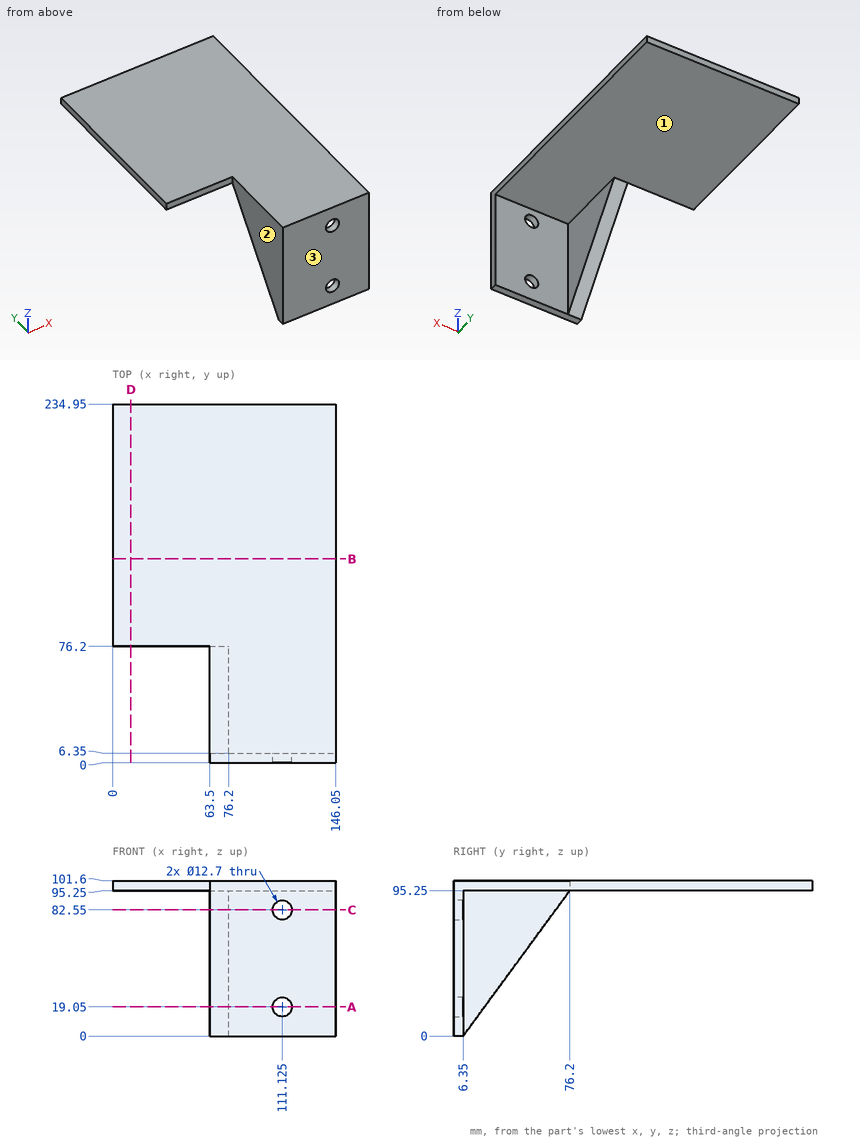
Geometry: see drawing. Coordinates: mm, zero at the bounding-box minimum. A direction names the side the tool comes from. Give positions to 0.01 mm unless a question says otherwise; leave off trailing zeros. Write each loop counter-clockwise with the first axis right and the second up, starting at its lowest first coordinate (ties: lowest second). Pieces come first, ordered by that corner, then holes. Notation, with made-up numbers: (84.5, 48.5) -> (131.5, 48.5) arc R10 cw to (131.5, 64.5) -> close; hole circle Ø10 at (15.25, 37.25). An arc over 180 degrees is marked (long way). Use one line per item in the form item = value. Start each with the question number.
1) Ray query, probe 1 along X at (y, z) = (1, 19); probe 2 along Z at (x, y) = (17, 101); probe 3 along Y at (x, z) = (26, 98.5). Return the intervals inside material, ascending. Write a range as from..to.
2) Set-up query: the marked faces 1, 2 and 3. Return all of +Z, -Z, +X, -X, +Y, -Y with unobstructed straight access to the full face (end or side cutting, diameter ignored); none if empty.
3) Section query D-D on x = 12. Return the cut outline in (y, z).
4) Section query C-C on z = 82.55. Return the cut outline in (x, y) (3 decimals).
5) Section query B-B on y = 133.5. Return the cut outline in (x, z).
6) Pin query (flat end, axial travel): pin 1 (2 mm diameter, centred on x = 123, y = 83, fed in from -Z); pin 2 (20.5 mm diameter, centred on x = 111.125, z = 19.05, fed in from +Y); pin 3 (21 mm diameter, centred on y = 54.5, z = 56.5, fed in from +X). Return the tip coordinate at first contact, or that it passes through.
7) Section query A-A on z = 19.05. Return the cut outline in (x, y) (3 decimals), then the cut area to 3 significant figures.
Outcome:
q1.probe_1 = 63.5..104.78, 117.47..146.05
q1.probe_2 = 95.25..101.6
q1.probe_3 = 76.2..234.95
q2.face_1 = -Z, +X, +Y
q2.face_2 = +Z, -Z, -X, -Y
q2.face_3 = +Z, -Z, +X, -X, -Y
q3.outline = (76.2, 95.25) -> (234.95, 95.25) -> (234.95, 101.6) -> (76.2, 101.6) -> close
q4.outline = (63.5, 0) -> (104.775, 0) -> (104.775, 6.35) -> (76.2, 6.35) -> (76.2, 66.887) -> (63.5, 66.887) -> close; (117.475, 0) -> (146.05, 0) -> (146.05, 6.35) -> (117.475, 6.35) -> close
q5.outline = (0, 95.25) -> (146.05, 95.25) -> (146.05, 101.6) -> (0, 101.6) -> close
q6.pin_1 = 95.25
q6.pin_2 = 6.35
q6.pin_3 = 76.2
q7.outline = (63.5, 0) -> (104.775, 0) -> (104.775, 6.35) -> (76.2, 6.35) -> (76.2, 20.32) -> (63.5, 20.32) -> close; (117.475, 0) -> (146.05, 0) -> (146.05, 6.35) -> (117.475, 6.35) -> close
q7.area = 621 mm^2
